```python
from build123d import *

# Parameters (mm, degrees)
SKETCH1_R           = 15
SKETCH1_R_2         = 8
BOSS_EXTRUDE1_DEPTH = 28
SKETCH2_R           = 15
SKETCH2_R_2         = 8
BOSS_EXTRUDE2_DEPTH = 28
SKETCH3_R           = 8
CUT_EXTRUDE1_DEPTH  = 70.426219995
SKETCH4_R           = 8
CUT_EXTRUDE2_DEPTH  = 70.426219995


with BuildPart() as part:
    # Sketch1 → Boss-Extrude1 (new, symmetric)
    with BuildSketch(Plane(origin=(0, 0, 0), x_dir=(1, 0, 0), z_dir=(0, 1, 0))):
        with Locations(Location((0, 0, 0), (0, 0, 270))):
            Circle(SKETCH1_R)
        with Locations(Location((0, 0, 0), (0, 0, 270))):
            Circle(SKETCH1_R_2, mode=Mode.SUBTRACT)
    extrude(amount=BOSS_EXTRUDE1_DEPTH, both=True)

    # Sketch2 → Boss-Extrude2 (add, symmetric)
    with BuildSketch(Plane(origin=(0, 0, 0), x_dir=(0, 0, -1), z_dir=(1, 0, 0))):
        with Locations((15, 0)):
            Circle(SKETCH2_R)
        with Locations((15, 0)):
            Circle(SKETCH2_R_2, mode=Mode.SUBTRACT)
    extrude(amount=BOSS_EXTRUDE2_DEPTH, both=True)

    # Sketch3 → Cut-Extrude1 (cut, through all)
    with BuildSketch(Plane(origin=(0, 28, 0), x_dir=(1, 0, 0), z_dir=(0, 1, 0))):
        with Locations(Location((0, 0, 0), (0, 0, 270))):
            Circle(SKETCH3_R)
    extrude(amount=-CUT_EXTRUDE1_DEPTH, mode=Mode.SUBTRACT)

    # Sketch4 → Cut-Extrude2 (cut, through all)
    with BuildSketch(Plane(origin=(28, 0, 0), x_dir=(0, 0, -1), z_dir=(1, 0, 0))):
        with Locations((15, 0)):
            Circle(SKETCH4_R)
    extrude(amount=-CUT_EXTRUDE2_DEPTH, mode=Mode.SUBTRACT)


solid = part.part
```
The listing builds one solid part. Answer for the finished solid, in the listing's coordinates (mm). A direction names the side the tool comes from. Give positions to 0.01 mm unless a question says otherwise; leave off trailing zeros. Write each loop counter-clockwise with the first axis right and the second up, starting at its lowest first coordinate (ties: lowest second). Pieces come first, ordered by that corner, then holes. Notation, with made-up numbers: (-27, 81.25) - (-18, 81.25) arc R19 ccw to (-18, 115.25) - close; hole circle Ø8 at (74, 56). An arc over 180 degrees is marked (long way). Use one line per item in the form item = value. Start each with the question number.
1) A tool of negligible diameter and unlimited length cuts with its end or side. For faces 5 (the face through (-5.745, 0.392, 13.856)), 6 (the face through (-28, -6, -21)), from which of +Z, -Z, +X, -X, +Y, -Y can it reach the whole face along a straight path? Write none if from no direction.
2) Flat-ended cylindrical pins translate along their axes: pin 1 Ø10 at (x, z) = (-3, -1) entering from -Y; pin 2 Ø3 at (x, y) = (-1, 21.5) entering from -Z; pin 3 Ø5 at (x, y) = (-19.5, 15) entering from +Z; pin 4 Ø5 at (y, z) = (14, 5) entering from -X. Find the tip coordinate at first contact, or state that the pin passes through.
3) The mould has two halves that part along Y. Classify faces 1 (the face through (-6, -28, 6)), 2 (the face through (0.392, -5.745, -28.856)), 3 (the face through (28, -6, -21)), 4 (the face through (-6, 28, 6)): pulls with the +Y half, pulls with the -Y half, needs draft (parallel to the pull), parting line crosses it, or undercut.
4) Find section C-C on x = 0. Determine the outline of the cut face in (y, z), plus the area to 3 significant figures.
5) Find section A-A on z = -2.5. Determine the outline of the cut face in (x, y).
6) Find section D-D on y = 11. Determine the outline of the cut face in (x, z).
7) Find section B-B on y = 5. Determine the outline of the cut face in (x, z) (3 decimals), plus the area to 3 significant figures.
8) Consider line 1 along X through (y, z) = (7, 0); line 2 along X through (y, z) = (22, -1.5). Determine where each line is inside the solid, lowest interval first. Write a range as from..to.
Geometry results:
q1.face_5 = none
q1.face_6 = +Z, -Z, -X, +Y, -Y
q2.pin_1 = -28
q2.pin_2 = -15
q2.pin_3 = -6.71
q2.pin_4 = -14.79
q3.face_1 = pulls with the -Y half
q3.face_2 = parting line crosses it
q3.face_3 = needs draft
q3.face_4 = pulls with the +Y half
q4.outline = (-28, -15) - (-15, -15) arc R15 ccw to (15, -15) - (28, -15) - (28, -8) - (3.87, -8) arc R8 cw (long way) to (-3.87, -8) - (-28, -8) - close; (-28, 8) - (28, 8) - (28, 15) - (-28, 15) - close
q4.area = 942 mm2
q5.outline = (-28, -8.29) - (-14.79, -8.29) - (-14.79, -28) - (-7.6, -28) - (-7.6, 28) - (-14.79, 28) - (-14.79, 8.29) - (-28, 8.29) - close; (7.6, -28) - (14.79, -28) - (14.79, -8.29) - (28, -8.29) - (28, 8.29) - (14.79, 8.29) - (14.79, 28) - (7.6, 28) - close
q6.outline = (-28, -25.2) - (28, -25.2) - (28, -4.8) - (14.21, -4.8) arc R15 ccw (long way) to (-14.21, -4.8) - (-28, -4.8) - close; hole circle Ø16 at (0, 0)
q7.outline = (-28, -29.142) - (28, -29.142) - (28, -21.245) - (-28, -21.245) - close; (-28, -8.755) - (28, -8.755) - (28, -0.858) - (14.975, -0.858) arc R15 ccw (long way) to (-14.975, -0.858) - (-28, -0.858) - close; hole circle Ø16 at (0, 0)
q7.area = 1,060 mm2
q8.line_1 = -15..-8, 8..15
q8.line_2 = -14.92..-7.86, 7.86..14.92
